Build history of the part. All positions in model axes, mm. A direction names the side the tool comes from. Round coordinates to 2 decimals unless told otherwise and drop trailing zeros. Loops run counter-clockwise (first coordinate to the right, second up) from the corner with the lowest first, then second, coordinate; pieces in that order, holes last.
from build123d import *

# Parameters (mm, degrees)
SKETCH2_R                = 60
BOSS_EXTRUDE1_DEPTH      = 60
SKETCH3_W                = 10
SKETCH3_H                = 10.47851478
BOSS_EXTRUDE2_DEPTH      = 60
FILLET2_R                = 3
CIRPATTERN1_COUNT        = 18
FILLET2_OF_CIRPATTERN1_R = 3
SKETCH4_R                = 10
CUT_EXTRUDE1_DEPTH       = 60
SKETCH5_R                = 11.25
CUT_EXTRUDE2_DEPTH       = 60
SCALE1_SCALE             = 0.2


with BuildPart() as part:
    # Sketch2 → Boss-Extrude1 (new body)
    with BuildSketch(Plane.XY):
        Circle(SKETCH2_R)
    extrude(amount=BOSS_EXTRUDE1_DEPTH)

    # Sketch3 → Boss-Extrude2 (add)
    with BuildSketch(Plane.XY.offset(60)):
        with Locations((0, 64.76074261)):
            Rectangle(SKETCH3_W, SKETCH3_H)
    boss_extrude2 = extrude(amount=-BOSS_EXTRUDE2_DEPTH)

    # Fillet2
    fillet2_edges = [part.edges().sort_by_distance(p)[0] for p in [
        (5, 70, 30),
        (0, 70, 0),
        (-5, 70, 30),
        (0, 70, 60),
    ]]
    fillet(fillet2_edges, radius=FILLET2_R)

    # CirPattern1: Boss-Extrude2 ×18 about axis
    cirpattern1_axis = Axis((0, 0, 0), (0, 0, 1))
    for i in range(1, CIRPATTERN1_COUNT):
        add(boss_extrude2.rotate(cirpattern1_axis, i * 360 / CIRPATTERN1_COUNT))

    # Fillet2 of CirPattern1
    fillet2_of_cirpattern1_edges = [part.edges().sort_by_distance(p)[0] for p in [
        (-19.242946929, 67.488584172, 30),
        (-23.941410033, 65.778483455, 0),
        (-28.639873137, 64.068382738, 30),
        (-23.941410033, 65.778483455, 60),
        (-41.164910462, 56.837049067, 30),
        (-44.995132678, 53.623111018, 0),
        (-48.825354894, 50.40917297, 30),
        (-44.995132678, 53.623111018, 60),
        (-58.121778265, 39.330127019, 30),
        (-60.621778265, 35, 0),
        (-63.121778265, 30.669872981, 30),
        (-60.621778265, 35, 60),
        (-68.068301823, 17.079411202, 30),
        (-68.936542711, 12.155372437, 0),
        (-69.804783599, 7.231333672, 30),
        (-68.936542711, 12.155372437, 60),
        (-69.804783599, -7.231333672, 30),
        (-68.936542711, -12.155372437, 0),
        (-68.068301823, -17.079411202, 30),
        (-68.936542711, -12.155372437, 60),
        (-63.121778265, -30.669872981, 30),
        (-60.621778265, -35, 0),
        (-58.121778265, -39.330127019, 30),
        (-60.621778265, -35, 60),
        (-48.825354894, -50.40917297, 30),
        (-44.995132678, -53.623111018, 0),
        (-41.164910462, -56.837049067, 30),
        (-44.995132678, -53.623111018, 60),
        (-28.639873137, -64.068382738, 30),
        (-23.941410033, -65.778483455, 0),
        (-19.242946929, -67.488584172, 30),
        (-23.941410033, -65.778483455, 60),
        (-5, -70, 30),
        (0, -70, 0),
        (5, -70, 30),
        (0, -70, 60),
        (19.242946929, -67.488584172, 30),
        (23.941410033, -65.778483455, 0),
        (28.639873137, -64.068382738, 30),
        (23.941410033, -65.778483455, 60),
        (41.164910462, -56.837049067, 30),
        (44.995132678, -53.623111018, 0),
        (48.825354894, -50.40917297, 30),
        (44.995132678, -53.623111018, 60),
        (58.121778265, -39.330127019, 30),
        (60.621778265, -35, 0),
        (63.121778265, -30.669872981, 30),
        (60.621778265, -35, 60),
        (68.068301823, -17.079411202, 30),
        (68.936542711, -12.155372437, 0),
        (69.804783599, -7.231333672, 30),
        (68.936542711, -12.155372437, 60),
        (69.804783599, 7.231333672, 30),
        (68.936542711, 12.155372437, 0),
        (68.068301823, 17.079411202, 30),
        (68.936542711, 12.155372437, 60),
        (63.121778265, 30.669872981, 30),
        (60.621778265, 35, 0),
        (58.121778265, 39.330127019, 30),
        (60.621778265, 35, 60),
        (48.825354894, 50.40917297, 30),
        (44.995132678, 53.623111018, 0),
        (41.164910462, 56.837049067, 30),
        (44.995132678, 53.623111018, 60),
        (28.639873137, 64.068382738, 30),
        (23.941410033, 65.778483455, 0),
        (19.242946929, 67.488584172, 30),
        (23.941410033, 65.778483455, 60),
    ]]
    fillet(fillet2_of_cirpattern1_edges, radius=FILLET2_OF_CIRPATTERN1_R)

    # Sketch4 → Cut-Extrude1 (cut)
    with BuildSketch(Plane.XY.offset(60)):
        Circle(SKETCH4_R)
    extrude(amount=-CUT_EXTRUDE1_DEPTH, mode=Mode.SUBTRACT)

    # Sketch5 → Cut-Extrude2 (cut)
    with BuildSketch(Plane(origin=(0, 0, 0), x_dir=(-1, 0, 0), z_dir=(0, 0, -1))):
        Circle(SKETCH5_R)
    extrude(amount=-CUT_EXTRUDE2_DEPTH, mode=Mode.SUBTRACT)


with BuildPart() as part_1:
    # Scale1: scaled about (3e-09, 1e-09, 29.999999969)
    add(part.part.scale(SCALE1_SCALE).moved(Location((2e-09, 1e-09, 23.999999975))))


solid = part_1.part
(1) Probe line 1 (Y direction, x = 0, z = 28.5); line 2 (Y direction, x = 11, z = 31); line 3 (X direction, y = 12.75, z = 30). List the from-to ranges inside material, lowest first.
Responses:
line 1: y = -14 to -2.25, 2.25 to 14
line 2: y = -7.51 to -5.2, -4.8 to 4.8, 5.2 to 7.51
line 3: x = -5.48 to -3.58, -1 to 1, 3.58 to 5.48
(2) Slice it at C-C on y = -4.5. List the corners of the cut face in (x, z), plus the area to 3 significant figures.
Responses:
outline: (-11.12, 24) - (11.12, 24) - (11.12, 36) - (-11.12, 36) - close
area: 267 mm2
(3) Slice it at D-D on y = 8. List the corners of the cut face in (x, z), plus the area to 3 significant figures.
Responses:
outline: (-8.94, 24) - (8.94, 24) - (8.94, 36) - (-8.94, 36) - close
area: 215 mm2
(4) Slice it at B-B on y = 0. List the corners of the cut face in (x, z).
Responses:
outline: (-12, 24) - (-2.25, 24) - (-2.25, 36) - (-12, 36) - close; (2.25, 24) - (12, 24) - (12, 36) - (2.25, 36) - close
(5) Slice it at A-A on x = 0. List the corners of the cut face in (y, z), plus the area to 3 significant figures.
Responses:
outline: (-14, 24.6) arc R0.6 ccw to (-13.4, 24) - (-2.25, 24) - (-2.25, 36) - (-13.4, 36) arc R0.6 ccw to (-14, 35.4) - close; (2.25, 24) - (13.4, 24) arc R0.6 ccw to (14, 24.6) - (14, 35.4) arc R0.6 ccw to (13.4, 36) - (2.25, 36) - close
area: 282 mm2
(6) Pull direction X, two halves, no side cores. Call faces 1 (the face through (9.517, 10.067, 29.916)), 2 (the face through (-4.7, -12.9, 24.1)), 3 (the face through (-2.07, 11.82, 29.92)): +X half, -X half, draft (parallel to the pull), parting line (faces both ways), or undercut.
Responses:
face 1: +X half
face 2: -X half
face 3: undercut
(7) Which spindle directions (+Z, -Z, +X, -X, +Y, -Y) get a long thin tool onto all of the face, cutting with end or side? Do faces 4 (the face through (-7.38, 10.35, 30.08)), 5 (the face through (-10.47, -7.2, 30.08)), 6 (the face through (-5.27, -11.56, 30.08)). Say none if no direction does.
Responses:
face 4: +Z, -Z, +Y
face 5: +Z, -Z, -Y
face 6: +Z, -Z
(8) Pin check, flat tips, straight feed: P1, Ø1.2, axis at y = 12.5, z = 27.5, coming from the -X side; P2, Ø3, axis at x = 10, z = 33, coming from the +Y side; P3, Ø1.5, axis at x = 4, z = 26, coming from the +Y side. Stop position of each tip, or through.
Responses:
P1: stops at x = -5.56
P2: stops at y = 11.09
P3: stops at y = 13.33
